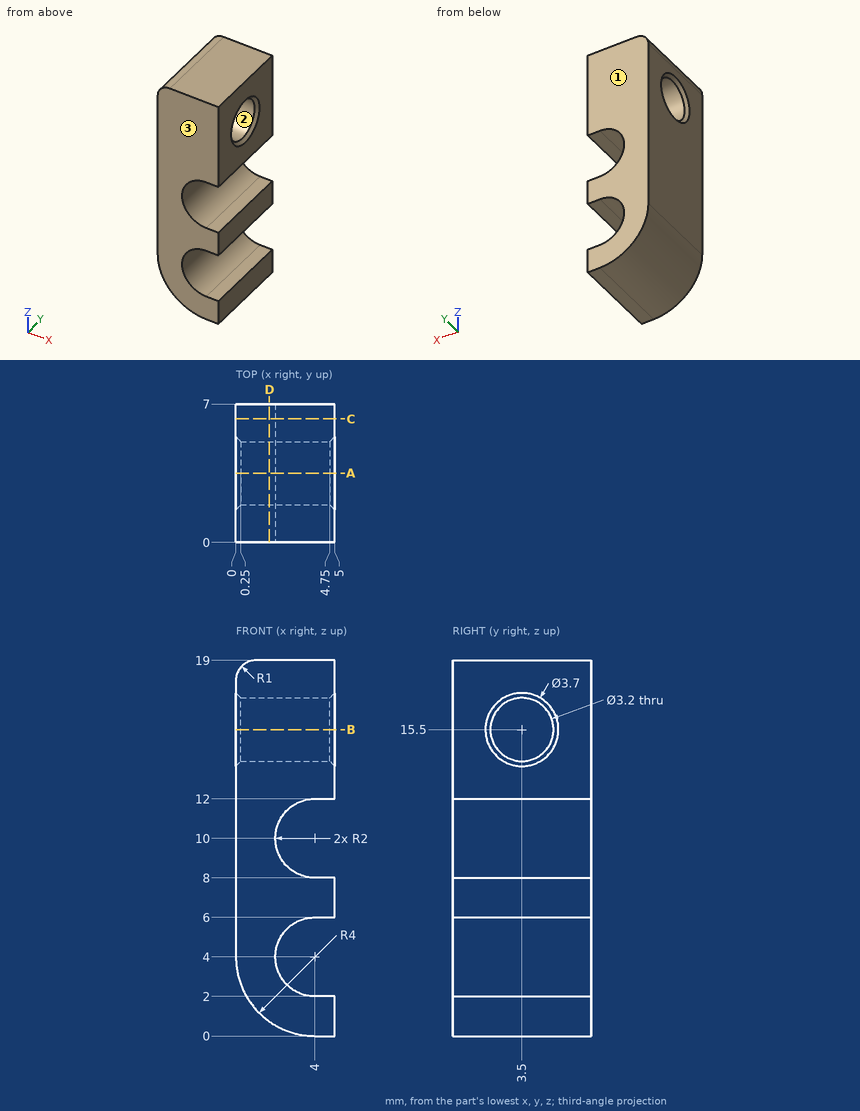
The drawing under review shows one solid part. Ordinate dimensions are in mm from its lowest x, y, z. Coordinates: 2 decimals unless noted, no trailing zeros. Write each loop counter-clockwise with the first axis right and the second up, starting at its lowest first coordinate (ties: lowest second). Pieces come first, ordered by that corner, then holes. Notation, with made-up numbers: M -3.75,-5 L 5.25,-5 A26 cw 5.25,15 Z; hole C 11,-4.5 d5. An arc over 180 degrees is marked long. Answer as a JSON object with one key per item and string values.
Item 1: Insertion check: pin 1 Ø1.5 at (y, z) = (2.5, 2.5) entering from -X. The pin has a flat end and moves straight along its axis. Give the tip position at first contact, or say it passes through.
Outcome:
{"pin 1": "x = 0.07"}
Item 2: Add section B-B, the plane z = 15.5. Give the boundary of the cut face in (x, y).
Outcome:
{"outline": "M 0,0 L 5,0 L 5,1.65 L 4.75,1.9 L 0.25,1.9 L 0,1.65 Z; M 0,5.35 L 0.25,5.1 L 4.75,5.1 L 5,5.35 L 5,7 L 0,7 Z"}
Item 3: Add section A-A, the plane y = 3.5. Give the boundary of the cut face in (x, z), and give its area (3 significant figures).
Outcome:
{"outline": "M 0,4 A4 ccw 4,0 L 5,0 L 5,2 L 4,2 A2 cw 4,6 L 5,6 L 5,8 L 4,8 A2 cw 4,12 L 5,12 L 5,13.65 L 4.75,13.9 L 0.25,13.9 L 0,13.65 Z; M 0,17.35 L 0.25,17.1 L 4.75,17.1 L 5,17.35 L 5,19 L 1,19 A1 ccw 0,18 Z", "area": "54.7 mm²"}
Item 4: Draft analysis for pull direction Y (two halves, no side actions). For the marked faces 1, 2 and 3, state which applies: pulls with the +Y half, pulls with the -Y half, needs draft (parallel to the pull), parting line crosses it, or undercut.
Outcome:
{"face 1": "pulls with the +Y half", "face 2": "undercut", "face 3": "pulls with the -Y half"}
Item 5: Wall thickness on probe 1 along Z at (x, y) = (4.3, 5.5); probe 2 along Y at (x, z) = (1.75, 15.5); probe 3 along Z at (x, y) = (3.65, 2.5): over which ranges is each line inside the solid? List them lowest first.
Outcome:
{"probe 1": "0 to 2, 6 to 8, 12 to 19", "probe 2": "0 to 1.9, 5.1 to 7", "probe 3": "0.02 to 2.03, 5.97 to 8.03, 11.97 to 14.25, 16.75 to 19"}
Item 6: Add section D-D, the plane x = 1.7. Give the boundary of the cut face in (y, z).
Outcome:
{"outline": "M 0,0.73 L 7,0.73 L 7,19 L 0,19 Z; hole C 3.5,15.5 d3.2"}
Item 7: Add section C-C, the plane y = 6.25. Give the boundary of the cut face in (x, z), and give its area (3 significant figures).
Outcome:
{"outline": "M 0,4 A4 ccw 4,0 L 5,0 L 5,2 L 4,2 A2 cw 4,6 L 5,6 L 5,8 L 4,8 A2 cw 4,12 L 5,12 L 5,19 L 1,19 A1 ccw 0,18 Z", "area": "70.8 mm²"}
